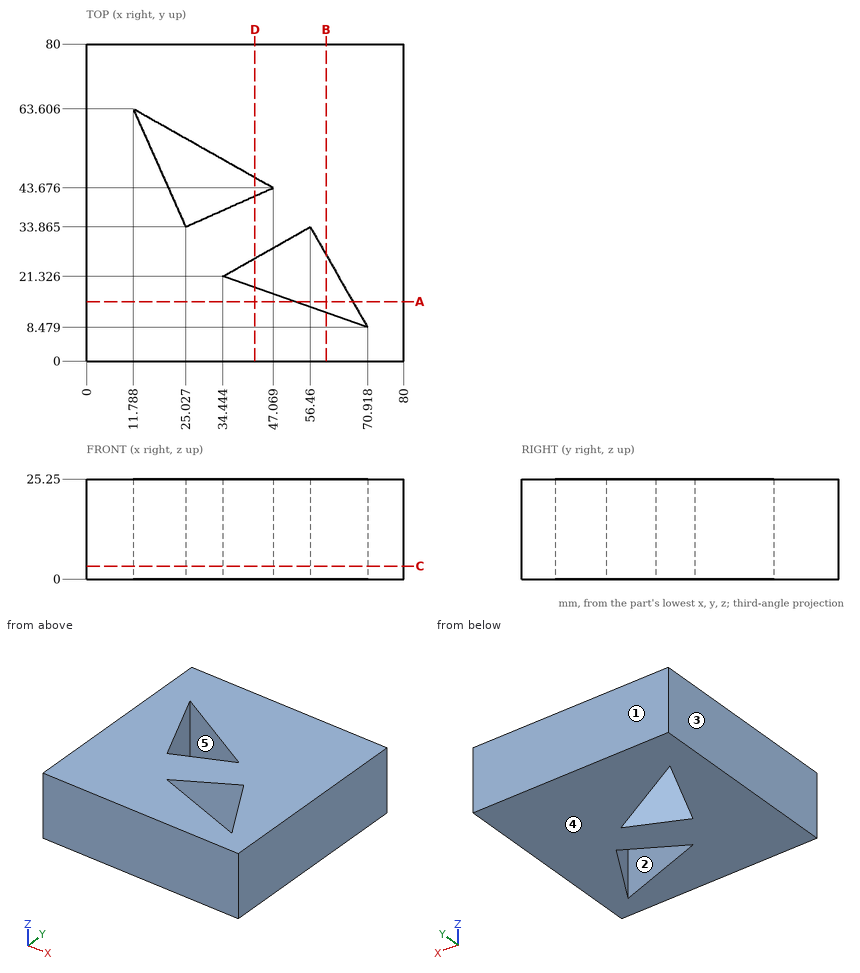
Source: three-view drawing plus pictorial views. Frame: mm from the lowest corner of the part. A direction names the side the tool comes from. Give positions to 0.01 mm unless a question says otherwise; leave off trailing zeros. Write each loop counter-clockwise with the first axis right and the second up, starting at its lowest first coordinate (ties: lowest second). Pieces come first, ordered by that corner, then holes.
(1) Access query for the marked faces 4 and 5. Directions: +Z, -Z, +X, -X, +Y, -Y. A direction counts if a zero-diameter tool reaches every point of the face in a straight line with its end or side. Return the directions, or none.
(2) Mould query, pull axis Y, two halves, no side actions, for the marked faces 1, 2 and 3. Classes: released by +Y, released by -Y, zero draft, split by the parting line, or undercut.
(3) First-contact query: P1, Ø12, axis at x = 27, z = 16, coming from the -Y side. Flat tip, straight axial feed; report the tip coordinate or a pass-through.
(4) Cut plane C-C, the plane z = 3.25. Return loops of the section in (x, y) (1 decimal), then the cut area to 3 significant figures.
(5) Cut plane A-A, the plane y = 15. Return loops of the section in (x, z).
(6) Cut plane D-D, the plane x = 42.5. Return loops of the section in (y, z).
(7) Cut plane B-B, the plane x = 60.5. Return loops of the section in (y, z), then the cut area to 3 significant figures.
(8) Ray query, line 1 (Y direction, x = 44.5, z = 23.5) (1 decimal); line 2 (X direction, y = 30, z = 18.5) (1 decimal); line 3 (Y direction, x = 25.5, z = 15.5) (1 decimal). Return the intervals inside material, ascending.
Values follow:
1. face 4: -Z, +X, -X, +Y, -Y
1. face 5: +Z, -Z
2. face 1: released by +Y
2. face 2: undercut
2. face 3: zero draft
3. P1: stops at y = 0
4. outline: (0, 0) - (80, 0) - (80, 80) - (0, 80) - close; hole (11.8, 63.6) - (25, 33.9) - (47.1, 43.7) - close; hole (34.4, 21.3) - (70.9, 8.5) - (56.5, 33.9) - close
4. area: 5,640 mm2
5. outline: (0, 0) - (52.4, 0) - (52.4, 25.25) - (0, 25.25) - close; (67.2, 0) - (80, 0) - (80, 25.25) - (67.2, 25.25) - close
6. outline: (0, 0) - (18.49, 0) - (18.49, 25.25) - (0, 25.25) - close; (25.91, 0) - (41.64, 0) - (41.64, 25.25) - (25.91, 25.25) - close; (46.26, 0) - (80, 0) - (80, 25.25) - (46.26, 25.25) - close
7. outline: (0, 0) - (12.15, 0) - (12.15, 25.25) - (0, 25.25) - close; (26.77, 0) - (80, 0) - (80, 25.25) - (26.77, 25.25) - close
7. area: 1,650 mm2
8. line 1: y = 0 to 17.8, 27.1 to 42.5, 45.1 to 80
8. line 2: x = 0 to 49.7, 58.7 to 80
8. line 3: y = 0 to 34.1, 55.9 to 80
